Check sheet for the modelled part. Datum: model origin and axes. Units: mm. A direction names the side the tool comes from. Give positions to 0.01 mm unless a question says otherwise; leave off trailing zeros. Order: outer loops, then holes, each group sorted by start corner. A loop starts at its lowest first (then second) coordinate and runs counter-clockwise, first axis right, second up. Notation, with made-up numbers: (57, 47.5) -> (62, 47.5) arc R32 ccw to (62, 73.5) -> close; hole circle Ø3 at (-19.5, -21.5). An arc over 180 degrees is marked (long way). One line per question, with ' | ' between items.
```python
from build123d import *

# Parameters (mm, degrees)
CROQUIS1_R                 = 7.5
SALIENTE_EXTRUIR1_DEPTH    = 58.52
CROQUIS2_W                 = 10
CROQUIS2_H                 = 15.856290926
CORTAR_EXTRUIR1_DEPTH      = 10
CORTAR_EXTRUIR2_DEPTH      = 60.473442813
CORTAR_EXTRUIR2_DEPTH_BACK = 60.473442813
CORTAR_EXTRUIR3_DEPTH      = 60.473442936
CORTAR_EXTRUIR3_DEPTH_BACK = 60.473442936
CROQUIS4_R                 = 1.5
REDONDEO1_R                = 0.3
CROQUIS6_W                 = 40
CROQUIS6_H                 = 40
SALIENTE_EXTRUIR2_DEPTH    = 5


with BuildPart() as part:
    # Croquis1 → Saliente-Extruir1 (new body)
    with BuildSketch(Plane(origin=(0, 0, 0), x_dir=(1, 0, 0), z_dir=(0, 1, 0))):
        with Locations(Location((0, 0, 0), (0, 0, 270))):
            Circle(CROQUIS1_R)
    extrude(amount=SALIENTE_EXTRUIR1_DEPTH)

    # Croquis2 → Cortar-Extruir1 (cut)
    with BuildSketch(Plane(origin=(0, 58.52, 0), x_dir=(1, 0, 0), z_dir=(0, 1, 0))):
        Rectangle(CROQUIS2_W, CROQUIS2_H)
    extrude(amount=-CORTAR_EXTRUIR1_DEPTH, mode=Mode.SUBTRACT)

    # Croquis3 → Cortar-Extruir2 (cut, two sides: drawn at the far end of the back side and taken through both)
    with BuildSketch(Plane(origin=(0, 0, 0), x_dir=(0, 0, -1), z_dir=(1, 0, 0)).offset(-CORTAR_EXTRUIR2_DEPTH_BACK)):
        with BuildLine():
            Line((-119.071460559, 48.52), (-7.5, 48.52))
            Line((-7.5, 48.52), (-5.590169944, 48.52))
            Line((-5.590169944, 48.52), (-3.884856087, 55.472834289))
            ThreePointArc((-3.884856087, 55.472834289), (0.002300645, 58.519999338), (3.885949583, 55.468364822))
            Line((3.885949583, 55.468364822), (5.590169944, 48.52))
            Line((5.590169944, 48.52), (7.5, 48.52))
            Line((7.5, 48.52), (119.071460559, 48.52))
            Line((119.071460559, 48.52), (119.071460559, 271.662921117))
            Line((119.071460559, 271.662921117), (-119.071460559, 271.662921117))
            Line((-119.071460559, 271.662921117), (-119.071460559, 48.52))
        make_face()
    extrude(amount=CORTAR_EXTRUIR2_DEPTH + CORTAR_EXTRUIR2_DEPTH_BACK, mode=Mode.SUBTRACT)

    # Croquis4 → Cortar-Extruir3 (cut, two sides: drawn at the far end of the back side and taken through both)
    with BuildSketch(Plane(origin=(0, 0, 0), x_dir=(0, 0, -1), z_dir=(1, 0, 0)).offset(-CORTAR_EXTRUIR3_DEPTH_BACK)):
        with Locations((0, 54.52)):
            Circle(CROQUIS4_R)
    extrude(amount=CORTAR_EXTRUIR3_DEPTH + CORTAR_EXTRUIR3_DEPTH_BACK, mode=Mode.SUBTRACT)

    # Redondeo1
    # the kernel refuses this fillet: 0.3 mm, written as the material it takes off along each edge
    with BuildSketch(Plane(origin=(0, 48.52, 0), x_dir=(0.7377533967735658, 0, 0.6750703115595187), z_dir=(0.6750703115595187, 0, -0.7377533967735658))) as redondeo1_piece_1_section:
        with BuildLine():
            CenterArc((7.5 - REDONDEO1_R, REDONDEO1_R), REDONDEO1_R, 270, 90)
            Line((7.5 - REDONDEO1_R, 0), (7.5, 0))
            Line((7.5, 0), (7.5, REDONDEO1_R))
        make_face()
    redondeo1_piece_1 = revolve(axis=Axis((0, 48.52, 0), (0, -1, 0)), revolution_arc=47.540389462, mode=Mode.PRIVATE)
    redondeo1_piece_1 = split(redondeo1_piece_1, bisect_by=Plane(origin=(5, 48.469281218, 5.527384127), z_dir=(-1, 0, 0)), keep=Keep.TOP, mode=Mode.PRIVATE)
    add(redondeo1_piece_1, mode=Mode.SUBTRACT)
    with BuildSketch(Plane(origin=(0, 48.52, 0), x_dir=(-0.7377709544179419, 0, -0.675051123113827), z_dir=(-0.675051123113827, 0, 0.7377709544179419))) as redondeo1_piece_2_section:
        with BuildLine():
            CenterArc((7.5 - REDONDEO1_R, REDONDEO1_R), REDONDEO1_R, 270, 90)
            Line((7.5 - REDONDEO1_R, 0), (7.5, 0))
            Line((7.5, 0), (7.5, REDONDEO1_R))
        make_face()
    redondeo1_piece_2 = revolve(axis=Axis((0, 48.52, 0), (0, -1, 0)), revolution_arc=95.083759333, mode=Mode.PRIVATE)
    redondeo1_piece_2 = split(redondeo1_piece_2, bisect_by=Plane(origin=(-5, 48.469281136, -5.527384204), z_dir=(1, 0, 0)), keep=Keep.TOP, mode=Mode.PRIVATE)
    redondeo1_piece_2 = split(redondeo1_piece_2, bisect_by=Plane(origin=(5, 48.469281136, -5.527384204), z_dir=(-1, 0, 0)), keep=Keep.TOP, mode=Mode.PRIVATE)
    add(redondeo1_piece_2, mode=Mode.SUBTRACT)
    with BuildSketch(Plane(origin=(0, 48.52, 0), x_dir=(0, 0, 1), z_dir=(1, 0, 0))) as redondeo1_piece_3_section:
        with BuildLine():
            CenterArc((7.5 - REDONDEO1_R, REDONDEO1_R), REDONDEO1_R, 270, 90)
            Line((7.5 - REDONDEO1_R, 0), (7.5, 0))
            Line((7.5, 0), (7.5, REDONDEO1_R))
        make_face()
    redondeo1_piece_3 = revolve(axis=Axis((0, 48.52, 0), (0, -1, 0)), revolution_arc=47.540389462, mode=Mode.PRIVATE)
    redondeo1_piece_3 = split(redondeo1_piece_3, bisect_by=Plane(origin=(-5, 48.435444693, 6.94366102), z_dir=(1, 0, 0)), keep=Keep.TOP, mode=Mode.PRIVATE)
    add(redondeo1_piece_3, mode=Mode.SUBTRACT)

    # Croquis6 → Saliente-Extruir2 (add)
    with BuildSketch(Plane.XZ):
        Rectangle(CROQUIS6_W, CROQUIS6_H)
    extrude(amount=SALIENTE_EXTRUIR2_DEPTH)


solid = part.part
```
Q1. Section check C-C (x = -16.5). Enter the section's corners in (y, z), and give its area (3 significant figures).
Result sheet:
outline: (-5, -20) -> (0, -20) -> (0, 20) -> (-5, 20) -> close | area: 200 mm2
Q2. Mould release check, pull along Y, two halves, no side actions. Record for faces 4 (the face through (0, -5, 0)), 5 (the face through (-5.56, 52.81, -4.54)), 6 (the face through (0, -2, 20)), 7 (the face through (-6.27, 54.59, 1.5)): pulls with the +Y half, pulls with the -Y half, needs draft (parallel to the pull), parting line crosses it, or undercut.
Result sheet:
face 4: pulls with the -Y half | face 5: pulls with the +Y half | face 6: needs draft | face 7: undercut
Q3. Section check B-B (y = 54.52). Enter the section's corners in (x, z).
Result sheet:
outline: (-7.35, -1.5) arc R7.5 ccw to (-6.27, -4.12) -> (-5, -4.12) -> (-5, -1.5) -> close; (-7.35, 1.5) -> (-5, 1.5) -> (-5, 4.12) -> (-6.27, 4.12) arc R7.5 ccw to start; (5, -4.12) -> (6.27, -4.12) arc R7.5 ccw to (7.35, -1.5) -> (5, -1.5) -> close; (5, 1.5) -> (7.35, 1.5) arc R7.5 ccw to (6.27, 4.12) -> (5, 4.12) -> close
Q4. Depth check by flat-ended pin: pin 1 Ø5 at (y, z) = (54.52, 0) entering from +X; pin 2 Ø8 at (x, z) = (-4, -12) entering from +Y; pin 3 Ø4 at (y, z) = (22.5, -5) entering from +X; pin 4 Ø2.5 at (y, z) = (54.52, 0) entering from +X. Enter the tip coordinate at first touch or a pass-through.
Result sheet:
pin 1: stops at x = 7.5 | pin 2: stops at y = 0 | pin 3: stops at x = 6.87 | pin 4: passes through
Q5. Access from +Z, -Z, +X, -X, +Y, -Y to the whole of each face (thin tool, end or side, straight path). Record for faces 1 (the face through (5.95, 58.52, 0.07)), 2 (the face through (9, 0, 0)), 3 (the face through (0, 48.52, 0)).
Result sheet:
face 1: +X, -X, +Y | face 2: +Y | face 3: +Z, -Z, +Y
Q6. Section check D-D (y = 41.5). Enter the section's corners in (x, z).
Result sheet:
outline: circle Ø15 at (0, 0)
Q7. Thickness scan on line 1 (Y direction, x = 6, z = 0); line 2 (X direction, y = 43, z = 5); line 3 (X direction, y = 44, z = 0.5). Record the ranges inside material, lowest first.
Result sheet:
line 1: y = -5 to 53.02, 56.02 to 58.52 | line 2: x = -5.59 to 5.59 | line 3: x = -7.48 to 7.48
Q8. Section check A-A (z = 0). Enter the section's corners in (x, y).
Result sheet:
outline: (-20, -5) -> (20, -5) -> (20, 0) -> (7.5, 0) -> (7.5, 53.02) -> (5, 53.02) -> (5, 48.52) -> (-5, 48.52) -> (-5, 53.02) -> (-7.5, 53.02) -> (-7.5, 0) -> (-20, 0) -> close; (-7.5, 56.02) -> (-5, 56.02) -> (-5, 58.52) -> (-7.5, 58.52) -> close; (5, 56.02) -> (7.5, 56.02) -> (7.5, 58.52) -> (5, 58.52) -> close
